from build123d import *
from build123d.topology import SkipClean

# Parameters (mm, degrees)
SKETCH_2_R               = 4.5
EXTRUDE_1_DEPTH          = 8
EXTRUDE_2_DEPTH          = 4
EXTRUDE_2_DEPTH_BACK     = 11.5
CUT_EXTRUDE_1_DEPTH      = 41.717122437
CUT_EXTRUDE_1_DEPTH_BACK = 41.717122437
CUT_EXTRUDE_2_DEPTH      = 41.717122437
CUT_EXTRUDE_2_DEPTH_BACK = 41.717122437
SKETCH_6_R               = 1


with BuildPart() as part:
    # Эскиз2 → Бобышка-Вытянуть1 (new body)
    with BuildSketch(Plane.XY):
        with BuildLine():
            Line((-18.858561718, 18.044523082), (33.641438282, 18.044523082))
            ThreePointArc((33.641438282, 18.044523082), (34.348545063, 17.751629864), (34.641438282, 17.044523082))
            Line((34.641438282, 17.044523082), (34.641438282, 7.044523082))
            ThreePointArc((34.641438282, 7.044523082), (34.348545063, 6.337416301), (33.641438282, 6.044523082))
            Line((33.641438282, 6.044523082), (29.641438282, 6.044523082))
            ThreePointArc((29.641438282, 6.044523082), (26.105904376, 4.580056988), (24.641438282, 1.044523082))
            Line((24.641438282, 1.044523082), (24.641438282, -12.955476918))
            ThreePointArc((24.641438282, -12.955476918), (24.348545063, -13.662583699), (23.641438282, -13.955476918))
            Line((23.641438282, -13.955476918), (-9.858561718, -13.955476918))
            ThreePointArc((-9.858561718, -13.955476918), (-10.565668499, -13.662583699), (-10.858561718, -12.955476918))
            Line((-10.858561718, -12.955476918), (-10.858561718, 6.044523082))
            Line((-10.858561718, 6.044523082), (-17.858561718, 6.044523082))
            ThreePointArc((-17.858561718, 6.044523082), (-18.565668499, 6.337416301), (-18.858561718, 7.044523082))
            Line((-18.858561718, 7.044523082), (-18.858561718, 18.044523082))
        make_face()
        with Locations((-0.858561718, -3.955476918)):
            Circle(SKETCH_2_R, mode=Mode.SUBTRACT)
    extrude(amount=EXTRUDE_1_DEPTH)

    # Эскиз3 → Бобышка-Вытянуть2 (add, two sides: drawn at the far end of the back side and taken through both)
    with SkipClean():  # the faces are left unmerged after this step: merging them gives an invalid solid
        with BuildSketch(Plane.XY.offset(8).offset(-EXTRUDE_2_DEPTH_BACK)):
            with BuildLine():
                Line((27.141438282, 14.544523082), (27.141438282, 18.044523082))
                Line((27.141438282, 18.044523082), (33.141438282, 18.044523082))
                Line((33.141438282, 18.044523082), (33.141438282, 14.544523082))
                ThreePointArc((33.141438282, 14.544523082), (30.141438282, 11.544523082), (27.141438282, 14.544523082))
            make_face()
            with BuildLine():
                Line((-0.358561718, 14.544523082), (-0.358561718, 18.044523082))
                Line((-0.358561718, 18.044523082), (-6.358561718, 18.044523082))
                Line((-6.358561718, 18.044523082), (-6.358561718, 14.544523082))
                ThreePointArc((-6.358561718, 14.544523082), (-3.358561718, 11.544523082), (-0.358561718, 14.544523082))
            make_face()
            with BuildLine():
                Line((-6.358561718, -10.455476918), (-6.358561718, -13.955476918))
                Line((-6.358561718, -13.955476918), (-0.358561718, -13.955476918))
                Line((-0.358561718, -13.955476918), (-0.358561718, -10.455476918))
                ThreePointArc((-0.358561718, -10.455476918), (-0.519059003, -9.487373446), (-0.983377938, -8.622855294))
                ThreePointArc((-0.983377938, -8.622855294), (-1.135599023, -8.491670945), (-1.327173883, -8.4310107))
                ThreePointArc((-1.327173883, -8.4310107), (-2.473967575, -8.155532145), (-3.509794913, -7.591541073))
                ThreePointArc((-3.509794913, -7.591541073), (-3.692643427, -7.508192328), (-3.893539312, -7.503562458))
                ThreePointArc((-3.893539312, -7.503562458), (-5.661270208, -8.532579726), (-6.358561718, -10.455476918))
            make_face()
        extrude(amount=EXTRUDE_2_DEPTH + EXTRUDE_2_DEPTH_BACK)
    add(part.part.scale(1), mode=Mode.REPLACE)  # the faces are merged on a copy

    # Эскиз5 → Вырез-Вытянуть1 (cut, two sides: drawn at the far end of the back side and taken through both)
    with BuildSketch(Plane.XY.offset(8).offset(-CUT_EXTRUDE_1_DEPTH_BACK)):
        with BuildLine():
            Line((14.520862779, 6.560547497), (2.520862779, 6.560547497))
            ThreePointArc((2.520862779, 6.560547497), (0.399542436, 5.681867841), (-0.479137221, 3.560547497))
            Line((-0.479137221, 3.560547497), (-0.479137221, -8.439452503))
            Line((-0.479137221, -8.439452503), (14.520862779, -8.439452503))
            ThreePointArc((14.520862779, -8.439452503), (16.642183123, -7.560772847), (17.520862779, -5.439452503))
            Line((17.520862779, -5.439452503), (17.520862779, 3.560547497))
            ThreePointArc((17.520862779, 3.560547497), (16.642183123, 5.681867841), (14.520862779, 6.560547497))
        make_face()
    extrude(amount=CUT_EXTRUDE_1_DEPTH + CUT_EXTRUDE_1_DEPTH_BACK, mode=Mode.SUBTRACT)

    # Эскиз6 → Вырез-Вытянуть2 (cut, two sides: drawn at the far end of the back side and taken through both)
    with BuildSketch(Plane.XY.offset(8).offset(-CUT_EXTRUDE_2_DEPTH_BACK)):
        with Locations((-3.358561718, 14.544523082)):
            Circle(SKETCH_6_R)
        with Locations((30.141438282, 14.544523082)):
            Circle(SKETCH_6_R)
        with Locations((-3.358561718, -10.455476918)):
            Circle(SKETCH_6_R)
    extrude(amount=CUT_EXTRUDE_2_DEPTH + CUT_EXTRUDE_2_DEPTH_BACK, mode=Mode.SUBTRACT)


solid = part.part
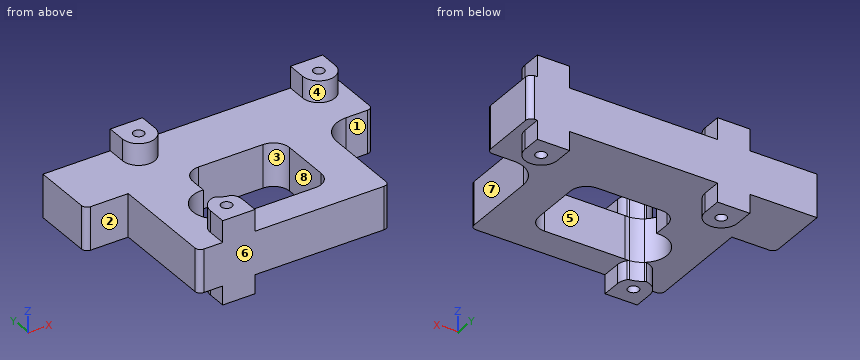
Input: part model. Units: mm. Frame: model coordinates. Face numbers are marked on the shaded views. A direction names the side the tool comes from. Coordinates: 2 decimals unless noted, no trailing zeros. Loops run counter-clockwise (first coordinate to the right, second up) from the corner with the lowest first, then second, coordinate; pieces in that order, holes last.
(1) Section A-A on z = 9.5. Return the cut outline in (x, y), then the cut area to 3 significant figures.
(2) Section C-C on y = -6. Return the cut outline in (x, z), then the cut area to 3 significant figures.
(3) Section B-B on x = 9.5. Return the cut outline in (y, z), then the cut area to 3 significant figures.
(4) Pull-direction query (Y, two-part tool) for the marked faces 5, 6, 7 and 8; classes: released by +Y, released by -Y, zero draft, split by the parting line, or undercut.
(5) Set-up query: the marked faces 1, 2, 3 and 4. Return all of +Z, -Z, +X, -X, +Y, -Y with unobstructed straight access to the full face (end or side cutting, diameter ignored); none if empty.
(6) First-contact query: pin 1 Ø1.5 at (y, z) = (2, 4.5) entering from +X; pin 2 Ø6.5 at (y, z) = (0, 3.5) entering from -X; pin 3 Ø7.5 at (x, z) = (-15.5, 4) entering from -Y; pin 4 Ø2.5 at (x, y) = (-3.36, -10.46) entering from +Z. Flat tips, straight axial feed; report the tip coordinate or a pass-through.
(7) Material intervals for probe 1 along X at (y, z) = (14, 3.5); probe 2 along Y at (x, z) = (11, 5.25); probe 3 along Y at (x, z) = (-5, 0.5), sorted ascending.
(8) Section D-D on z = 4.75. Return the cut outline in (x, y).
Data:
1. outline: (-6.36, -13.96) - (-0.36, -13.96) - (-0.36, -10.46) arc R3 ccw to (-0.98, -8.62) arc R0.5 ccw to (-1.33, -8.43) arc R4.5 cw to (-3.51, -7.59) arc R0.5 ccw to (-3.89, -7.5) arc R3 ccw to (-6.36, -10.46) - close; (-6.36, 14.54) arc R3 ccw to (-0.36, 14.54) - (-0.36, 18.04) - (-6.36, 18.04) - close; (27.14, 14.54) arc R3 ccw to (33.14, 14.54) - (33.14, 18.04) - (27.14, 18.04) - close; hole circle Ø2 at (-3.36, -10.46); hole circle Ø2 at (-3.36, 14.54); hole circle Ø2 at (30.14, 14.54)
1. area: 95.0 mm2
2. outline: (-10.86, 0) - (-4.87, 0) - (-4.87, 8) - (-10.86, 8) - close; (17.47, 0) - (24.64, 0) - (24.64, 8) - (17.47, 8) - close
2. area: 105 mm2
3. outline: (-13.96, 0) - (-8.44, 0) - (-8.44, 8) - (-13.96, 8) - close; (6.56, 0) - (18.04, 0) - (18.04, 8) - (6.56, 8) - close
3. area: 136 mm2
4. face 5: undercut
4. face 6: released by -Y
4. face 7: zero draft
4. face 8: undercut
5. face 1: +Z, -Z, +X, -Y
5. face 2: +Z, -Z, -X, -Y
5. face 3: +Z, -Z
5. face 4: +Z, -Y
6. pin 1: stops at x = 24.94
6. pin 2: stops at x = -10.86
6. pin 3: stops at y = 6.04
6. pin 4: stops at z = 12
7. probe 1: x = -18.86 to -4.2, -2.52 to 29.3, 30.98 to 34.64
7. probe 2: y = -13.96 to -8.44, 6.56 to 18.04
7. probe 3: y = -13.96 to -5.72, -2.2 to 18.04
8. outline: (-18.86, 7.04) arc R1 ccw to (-17.86, 6.04) - (-10.86, 6.04) - (-10.86, -12.96) arc R1 ccw to (-9.86, -13.96) - (23.64, -13.96) arc R1 ccw to (24.64, -12.96) - (24.64, 1.04) arc R5 cw to (29.64, 6.04) - (33.64, 6.04) arc R1 ccw to (34.64, 7.04) - (34.64, 17.04) arc R1 ccw to (33.64, 18.04) - (-18.86, 18.04) - close; hole circle Ø2 at (-3.36, -10.46); hole circle Ø2 at (-3.36, 14.54); hole (-0.48, -8.44) - (14.52, -8.44) arc R3 ccw to (17.52, -5.44) - (17.52, 3.56) arc R3 ccw to (14.52, 6.56) - (2.52, 6.56) arc R3 ccw to (-0.48, 3.56) - (-0.48, 0.53) arc R4.5 ccw (long way) to start; hole circle Ø2 at (30.14, 14.54)
